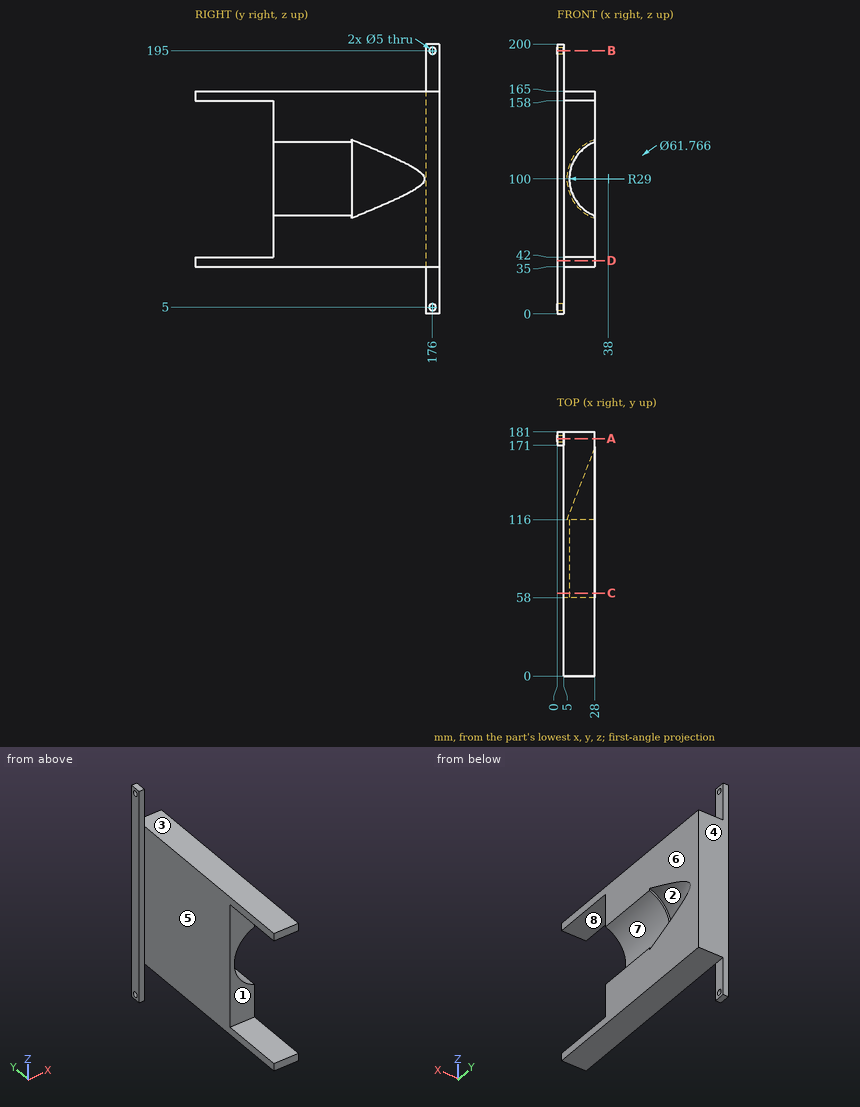
Source: three-view drawing plus pictorial views. Frame: mm from the lowest corner of the part. A direction names the side the tool comes from. Give positions to 0.01 mm unless a question says otherwise; leave off trailing zeros. Loops run counter-clockwise (first coordinate to the right, second up) from the corner with the lowest first, then second, coordinate; pieces in that order, holes last. Notation, with made-up numbers: (84, -5) -> (99, -5) arc R17 cw to (99, 21) -> close; hole circle Ø4 at (4, 52). An arc over 180 degrees is marked (long way). Use a Markdown table: item, result. Add a question column.
(1) Access query for the marked faces 5, 6, 7 and 8. Directions: +Z, -Z, +X, -X, +Y, -Y. A direction counts if a zero-diameter tool reaches every point of the face in a straight line with its end or side. Return the directions, or none.
(2) Section query D-D (z = 39.5). Output: boundary loops of the cut face in (x, y), then the cut area to 3 significant figures.
(3) First-contact query: pin 1 Ø1.5 at (y, z) = (130, 114.5) entering from -X; pin 2 Ø8 at (y, z) = (174, 14.5) entering from +X; pin 3 Ø2 at (x, z) = (8.5, 71.5) entering from -Y. Flat tips, straight axial feed; report the tip coordinate or a pass-through.
(4) Section query A-A (y = 176). Output: boundary loops of the cut face in (x, z), then the cut area to 3 significant figures.
(5) Section query C-C (y = 61.5). Output: boundary loops of the cut face in (x, z), then the cut area to 3 significant figures.
(6) Ray query, line 1 (Z direction, x = 1, y = 176); line 2 (Z direction, x = 8.75, y = 8); line 3 (Y direction, x = 1.2, z = 195). Return the intervals inside material, ascending.
(7) Pull-direction query (Y, two-part tool) for the marked faces 1, 2, 3 and 4; classes: +Y half, -Y half, draft (parallel to the pull), parting line (faces both ways), or undercut.
(8) Section query B-B (z = 195). Output: boundary loops of the cut face in (x, y), then the cut area to 3 significant figures.
Checked values:
| question | item | result |
|---|---|---|
| 1 | face 5 | +Z, -Z, -X, -Y |
| 1 | face 6 | +Z, -Z, +X, +Y, -Y |
| 1 | face 7 | +X, -Y |
| 1 | face 8 | +X, -X, -Y |
| 2 | outline | (0, 171) -> (5, 171) -> (5, 0) -> (28, 0) -> (28, 181) -> (0, 181) -> close |
| 2 | area | 4,210 mm^2 |
| 3 | pin 1 | x = 5 |
| 3 | pin 2 | x = 5 |
| 3 | pin 3 | y = 58 |
| 4 | outline | (0, 0) -> (5, 0) -> (5, 2.5) -> (0, 2.5) -> close; (0, 7.5) -> (5, 7.5) -> (5, 35) -> (28, 35) -> (28, 165) -> (5, 165) -> (5, 192.5) -> (0, 192.5) -> close; (0, 197.5) -> (5, 197.5) -> (5, 200) -> (0, 200) -> close |
| 4 | area | 3,940 mm^2 |
| 5 | outline | (5, 35) -> (28, 35) -> (28, 72.78) arc R29 cw to (28, 127.22) -> (28, 165) -> (5, 165) -> close |
| 5 | area | 2,240 mm^2 |
| 6 | line 1 | 0 to 2.5, 7.5 to 192.5, 197.5 to 200 |
| 6 | line 2 | 35 to 42, 158 to 165 |
| 6 | line 3 | 171 to 173.5, 178.5 to 181 |
| 7 | face 1 | -Y half |
| 7 | face 2 | undercut |
| 7 | face 3 | draft |
| 7 | face 4 | +Y half |
| 8 | outline | (0, 171) -> (5, 171) -> (5, 173.5) -> (0, 173.5) -> close; (0, 178.5) -> (5, 178.5) -> (5, 181) -> (0, 181) -> close |
| 8 | area | 25.0 mm^2 |
